Geometry: final body of the model. Coordinates: model frame, mm. A direction names the side the tool comes from. Round coordinates to 2 decimals unless told otherwise and drop trailing zeros. Loops run counter-clockwise (first coordinate to the right, second up) from the corner with the lowest first, then second, coordinate; pieces in that order, holes last. Notation, with made-up numbers: (-15, 88) - (31, 88) arc R28 ccw to (31, 114) - close; hole circle Ø8 at (35, 39.5). An arc over 180 degrees is marked (long way). Return JSON: item names as keys, results as strings. Group by question number.
1. First-contact query: pin 1 Ø1.5 at (x, y) = (9, -6.5) entering from +Z; pin 2 Ø2 at (y, z) = (-9.5, 6) entering from +X; pin 3 Ø6 at (x, z) = (4, 14.5) entering from -Y. Flat tips, straight axial feed; report the tip coordinate or a pass-through.
2. Draft query along Y for faces 1 (the face through (8.6, -0.6, 9.8)), 2 (the face through (9, -13.5, 5)), 3 (the face through (-9, 4, 12)). Return one class per face: +Y half, -Y half, draft (parallel to the pull), parting line (faces both ways), or undercut.
3. Set-up query: faces 4 (the face through (8.65, 7.51, 5.24)), 5 (the face through (9, 4, 12)). Return all of +Z, -Z, +X, -X, +Y, -Y with unobstructed straight access to the full face (end or side cutting, diameter ignored); none if empty.
4. Material intervals for probe 1 along X at (y, z) = (2.25, 4.5) (3 decimals); probe 2 along Z at (x, y) = (9, -9.5); probe 3 along Z at (x, y) = (-8.2, 8.5), sorted ascending.
5. Section A-A on z = 6. Return loops of the section in (x, y) (3 decimals), and give its area (3 significant figures).
6. Section B-B on y = 4.25. Return loops of the section in (x, z) (3 decimals).
7. Section C-C on x = -8. Return loops of the section in (y, z), and give its area (3 significant figures).
8. Section D-D on y = 8.5. Return loops of the section in (x, z) (3 decimals).
from build123d import *

# Parameters (mm, degrees)
F0_W     = 3
F0_H     = 24
F1_DEPTH = 12
F2_R     = 1.25
F3_DEPTH = 150
F4_DEPTH = 20
F5_R     = 5
F6_R     = 1
F7_DEPTH = 150


# Not quite as in the source:
# - a feature names something its author has since deleted; it is built from what else it names


with BuildPart() as f1:
    # F0 (on Top) → F1 (new body)
    with BuildSketch(Plane.XY):
        with Locations((8.625, -1.5)):
            Rectangle(F0_W, F0_H)
        with Locations((-8.625, -1.5)):
            Rectangle(F0_W, F0_H)
        Polygon((10.125, 13.5), (-10.125, 13.5), (-10.125, 10.5), (-7.125, 10.5), (7.125, 10.5), (10.125, 10.5), align=None)
    extrude(amount=F1_DEPTH)

    # F2 (on face) → F3 (cut)
    with BuildSketch(Plane.YZ.offset(10.125)):
        with Locations((-9.5, 6)):
            Circle(F2_R)
        with Locations((8.5, 6)):
            Circle(F2_R)
    extrude(amount=-F3_DEPTH, mode=Mode.SUBTRACT)

    # F0 (on Top) → F4 (join)
    with BuildSketch(Plane.XY):
        Polygon((10.125, 13.5), (-10.125, 13.5), (-10.125, 10.5), (-7.125, 10.5), (7.125, 10.5), (10.125, 10.5), align=None)
    extrude(amount=F4_DEPTH)

    # F5
    f5_edges = [f1.edges().sort_by_distance(p)[0] for p in [
        (8.625, 10.5, 12),
        (-8.625, 10.5, 12),
    ]]
    fillet(f5_edges, radius=F5_R)

    # F6
    f6_edges = [f1.edges().sort_by_distance(p)[0] for p in [
        (8.625, -13.5, 12),
        (-8.625, -13.5, 12),
    ]]
    fillet(f6_edges, radius=F6_R)

    # F2 (on face) → F7 (cut)
    with BuildSketch(Plane.YZ.offset(10.125)):
        with BuildLine():
            ThreePointArc((-4.4522145691, 12), (-0.5, 9.8), (3.4522145691, 12))
            Line((3.4522145691, 12), (-4.4522145691, 12))
        make_face()
    extrude(amount=-F7_DEPTH, mode=Mode.SUBTRACT)


solid = f1.part
Taken from the geometry:
{
 "1": {"pin 1": "z = 12", "pin 2": "through", "pin 3": "y = 10.5"},
 "2": {"face 1": "undercut", "face 2": "-Y half", "face 3": "draft"},
 "3": {"face 4": "+X, -X", "face 5": "+Z, +X, -X, -Y"},
 "4": {"probe 1": "-10.125 to -7.125, 7.125 to 10.125", "probe 2": "0 to 4.75, 7.25 to 12", "probe 3": "0 to 4.75, 7.25 to 13"},
 "5": {"outline": "(-10.125, -13.5) - (-7.125, -13.5) - (-7.125, -10.75) - (-10.125, -10.75) - close; (-10.125, -8.25) - (-7.125, -8.25) - (-7.125, 7.25) - (-10.125, 7.25) - close; (-10.125, 9.75) - (-7.125, 9.75) - (-7.125, 10.5) - (7.125, 10.5) - (7.125, 9.75) - (10.125, 9.75) - (10.125, 13.5) - (-10.125, 13.5) - close; (7.125, -13.5) - (10.125, -13.5) - (10.125, -10.75) - (7.125, -10.75) - close; (7.125, -8.25) - (10.125, -8.25) - (10.125, 7.25) - (7.125, 7.25) - close", "area": "175 mm2"},
 "6": {"outline": "(-10.125, 0) - (-7.125, 0) - (-7.125, 12) - (-10.125, 12) - close; (7.125, 0) - (10.125, 0) - (10.125, 12) - (7.125, 12) - close"},
 "7": {"outline": "(-13.5, 0) - (13.5, 0) - (13.5, 20) - (10.5, 20) - (10.5, 17) arc R5 cw to (5.5, 12) - (3.45, 12) arc R4.65 cw to (-4.45, 12) - (-12.5, 12) arc R1 ccw to (-13.5, 11) - close; hole circle Ø2.5 at (-9.5, 6); hole circle Ø2.5 at (8.5, 6)", "area": "331 mm2"},
 "8": {"outline": "(-10.125, 0) - (-7.125, 0) - (-7.125, 4.75) - (-10.125, 4.75) - close; (-10.125, 7.25) - (-7.125, 7.25) - (-7.125, 13) - (-10.125, 13) - close; (7.125, 0) - (10.125, 0) - (10.125, 4.75) - (7.125, 4.75) - close; (7.125, 7.25) - (10.125, 7.25) - (10.125, 13) - (7.125, 13) - close"}
}
